Can you work these out from the drawing? Everything is in mm from the part's minimum corner. Give positions to 0.01 mm unless a question says otherwise; leave off trailing zeros. Write each loop counter-clockwise with the first axis right and the second up, starting at its lowest first coordinate (ties: lowest second). Pieces come first, ordered by that corner, then holes. Notation, with made-up numbers: (45.5, -15.75) -> (94.5, -15.75) arc R28 ccw to (94.5, 6.25) -> close; hole circle Ø5 at (76.25, 88.25). An arc over 180 degrees is marked (long way). Use one line per item in the form item = value.
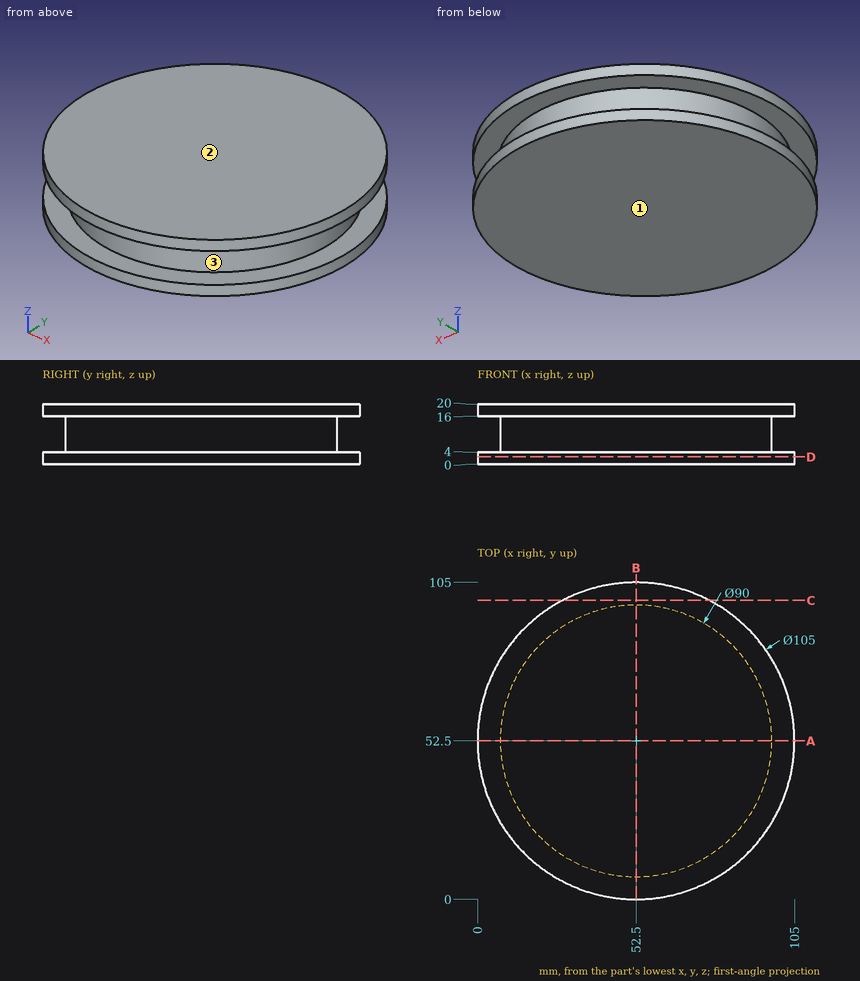
Q1. If I drill on line 1 along Z through (x, y) = (65, 8.5); line 2 along X through (y, z) = (61.5, 6.25); line 3 along X through (y, z) = (100.5, 16.25), over which ranges is the centre line in solid material (lowest first)? Write a range as from..to.
Result set:
line_1 = 0..4, 16..20
line_2 = 8.41..96.59
line_3 = 31.23..73.77
Q2. I want a section at A-A, the plane y = 52.5. Write out the boundary of the cut face in (x, z).
Result set:
outline = (0, 0) -> (105, 0) -> (105, 4) -> (97.5, 4) -> (97.5, 16) -> (105, 16) -> (105, 20) -> (0, 20) -> (0, 16) -> (7.5, 16) -> (7.5, 4) -> (0, 4) -> close
Q3. I want a section at D-D, the plane z = 2.5. Write out the boundary of the cut face in (x, y).
Result set:
outline = circle Ø105 at (52.5, 52.5)
Q4. Will these pins go through, and if not, where does the flat tip stop? pin 1 Ø8 at (y, z) = (91, 9.5) entering from +X; pin 2 Ø5 at (x, z) = (79, 9) entering from -Y; pin 3 Ø4 at (x, z) = (75.5, 3.5) entering from +Y.
Result set:
pin_1 = 81.39
pin_2 = 14.43
pin_3 = 100.62
Q5. I want a section at C-C, the plane y = 99. Write out the boundary of the cut face in (x, z), and give its area (3 significant figures).
Result set:
outline = (28.13, 0) -> (76.87, 0) -> (76.87, 4) -> (28.13, 4) -> close; (28.13, 16) -> (76.87, 16) -> (76.87, 20) -> (28.13, 20) -> close
area = 390 mm2
Q6. If we mould it in two halves opening along Z, with no side actions, what happens to the marked faces 1, 2 and 3? For each: +Z half, -Z half, draft (parallel to the pull), parting line (faces both ways), or undercut.
Result set:
face_1 = -Z half
face_2 = +Z half
face_3 = undercut
